The listing builds one solid part. Answer for the finished solid, in the listing's coordinates (mm). Coordinates: 2 decimals unless noted, no trailing zeros. Order: outer loops, then holes, each group sorted by start corner. A loop starts at its lowest first (then second) coordinate and runs counter-clockwise, first axis right, second up. Notation, with made-up numbers: (-28.5, -26.5) -> (-15.5, -26.5) arc R24 ccw to (-15.5, -2.5) -> close; hole circle Ø1 at (75, -1). An arc over 180 degrees is marked (long way). Return JSON: item names as keys, results as strings.
```python
from build123d import *

# Parameters (mm, degrees)
EXTRUDE_1_DEPTH          = 5
CUT_EXTRUDE_2_DEPTH      = 1
CUT_EXTRUDE_2_DEPTH_BACK = 6
CUT_EXTRUDE_3_REACH      = 7
CHAMFER_1_SIZE           = 5
CUT_EXTRUDE_6_DEPTH      = 1
CUT_EXTRUDE_6_DEPTH_BACK = 6
CHAMFER_2_SIZE           = 5
SKETCH_6_R               = 2.1
CUT_EXTRUDE_7_DEPTH      = 5
FILLET_1_R               = 10
M3X0_5_1_D               = 2.5
M3X0_5_1_DEPTH           = 8.5
M3X0_5_1_TIP             = 0.751075774
M4X0_7_2_D               = 3.3
M4X0_7_2_DEPTH           = 11.5
M4X0_7_2_TIP             = 0.991420021


with BuildPart() as part:
    # 草圖1 → 填料-伸長1 (new body)
    with BuildSketch(Plane.XY):
        Polygon((150, 0), (75, 129.903810568), (-75, 129.903810568), (-150, 0), (-75, -129.903810568), (75, -129.903810568), align=None)
    extrude(amount=EXTRUDE_1_DEPTH)

    # 草圖3 → 除料-伸長2 (cut, two sides)
    with BuildSketch(Plane.XY.offset(5)) as cut_extrude_2_sk:
        Polygon((-774.886138932, 69.903810568), (-109.641016151, 69.903810568), (-89.641016151, 69.903810568), (-89.641016151, 54.903810568), (0, 54.903810568), (0, 69.903810568), (109.641016151, 69.903810568), (774.886138932, 69.903810568), (774.886138932, 1400.394056128), (-774.886138932, 1400.394056128), align=None)
    extrude(amount=CUT_EXTRUDE_2_DEPTH, mode=Mode.SUBTRACT)
    extrude(cut_extrude_2_sk.sketch, amount=-CUT_EXTRUDE_2_DEPTH_BACK, mode=Mode.SUBTRACT)

    # 草圖4 → 除料-伸長3 (cut, up to next)
    with BuildSketch(Plane.XY.offset(5), mode=Mode.PRIVATE) as cut_extrude_3_sk1:
        Polygon((30, 0), (15, 25.980762114), (-15, 25.980762114), (-30, 0), (-15, -25.980762114), (15, -25.980762114), align=None)
    cut_extrude_3_tool1 = extrude(cut_extrude_3_sk1.sketch, amount=-CUT_EXTRUDE_3_REACH, mode=Mode.PRIVATE) & part.part
    add(cut_extrude_3_tool1.solids().sort_by_distance((0, 0, 5))[0], mode=Mode.SUBTRACT)

    # 導角1
    chamfer_1_edges = [part.edges().sort_by_distance(p)[0] for p in [
        (-89.641016151, 69.903810568, 2.5),
        (0, 69.903810568, 2.5),
    ]]
    chamfer(chamfer_1_edges, length=CHAMFER_1_SIZE)

    # 草圖5 → 除料-伸長6 (cut, two sides)
    with BuildSketch(Plane.XY.offset(5)) as cut_extrude_6_sk:
        Polygon((-692.345987228, -104.903810568), (-89.43375673, -104.903810568), (-30, -104.903810568), (-30, -64.903810568), (30, -64.903810568), (30, -104.903810568), (89.43375673, -104.903810568), (692.345987228, -104.903810568), (692.345987228, -1310.728271565), (-692.345987228, -1310.728271565), align=None)
    extrude(amount=CUT_EXTRUDE_6_DEPTH, mode=Mode.SUBTRACT)
    extrude(cut_extrude_6_sk.sketch, amount=-CUT_EXTRUDE_6_DEPTH_BACK, mode=Mode.SUBTRACT)

    # 導角2
    chamfer_2_edges = [part.edges().sort_by_distance(p)[0] for p in [
        (30, -104.903810568, 2.5),
        (-30, -104.903810568, 2.5),
        (-30, -64.903810568, 2.5),
        (30, -64.903810568, 2.5),
    ]]
    chamfer(chamfer_2_edges, length=CHAMFER_2_SIZE)

    # 草圖6 → 除料-伸長7 (cut)
    with BuildSketch(Plane.XY.offset(5)):
        with Locations((-50, -90)):
            Circle(SKETCH_6_R)
        with Locations((-120, 10)):
            Circle(SKETCH_6_R)
        with Locations((-60, 30)):
            Circle(SKETCH_6_R)
        with Locations((-20, -50)):
            Circle(SKETCH_6_R)
    cut_extrude_7 = extrude(amount=-CUT_EXTRUDE_7_DEPTH, mode=Mode.SUBTRACT)

    # 鏡射1: 除料-伸長7 across plane
    add(cut_extrude_7.mirror(Plane(origin=(0, 0, 0), x_dir=(0, 0, 1), z_dir=(1, 0, 0))), mode=Mode.SUBTRACT)

    # 圓角1
    fillet_1_edges = [part.edges().sort_by_distance(p)[0] for p in [
        (-150, 0, 2.5),
        (150, 0, 2.5),
        (109.641016151, 69.903810568, 2.5),
        (-109.641016151, 69.903810568, 2.5),
        (-89.43375673, -104.903810568, 2.5),
        (89.43375673, -104.903810568, 2.5),
    ]]
    fillet(fillet_1_edges, radius=FILLET_1_R)

    # M3x0.5 螺紋孔1
    with Locations(Plane.XY.offset(5)):
        with Locations((95, 15.096189432), (75, -54.903810568), (75, 15.096189432), (95, -54.903810568)):
            Hole(M3X0_5_1_D / 2, depth=M3X0_5_1_DEPTH)
            with Locations((0, 0, -(M3X0_5_1_DEPTH + M3X0_5_1_TIP / 2))):  # 118° drill point
                Cone(0, M3X0_5_1_D / 2, M3X0_5_1_TIP, mode=Mode.SUBTRACT)

    # M4x0.7 螺紋孔2
    with Locations(Plane.XY.offset(5)):
        with Locations((25, 35), (-25, -35), (-25, 35), (25, -35), (-35, 0), (35, 0)):
            Hole(M4X0_7_2_D / 2, depth=M4X0_7_2_DEPTH)
            with Locations((0, 0, -(M4X0_7_2_DEPTH + M4X0_7_2_TIP / 2))):  # 118° drill point
                Cone(0, M4X0_7_2_D / 2, M4X0_7_2_TIP, mode=Mode.SUBTRACT)


solid = part.part
```
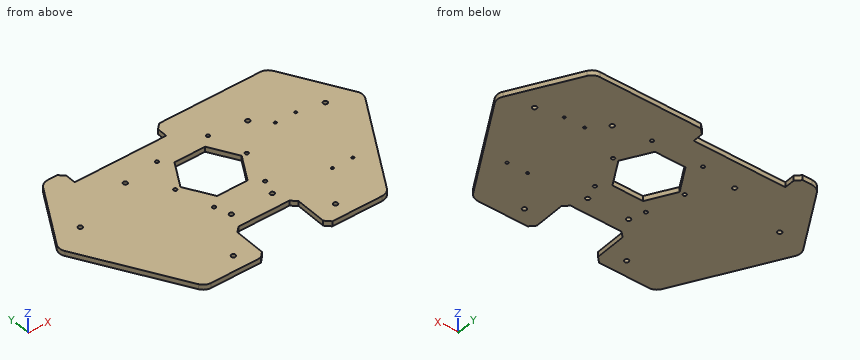
Item 1: The part is cut by section B-B on z = 2.6. Count the separate pieces of the cut face and the enclosed holes in it, plus the area to 3 significant figures.
Answer list:
{"separate pieces": "1", "enclosed holes": "19", "area": "36,900 mm2"}
Item 2: The part is cut by section A-A on x = -55. Determine the outline of the cut face in (y, z), plus the area to 3 significant figures.
Answer list:
{"outline": "(-104.9, 0) -> (54.9, 0) -> (54.9, 5) -> (-104.9, 5) -> close", "area": "799 mm2"}
Item 3: Flat-ended cylindrical pins translate along their axes: pin 1 (3 mm diameter, centred on x = 25, y = 35, fed in from -Z); pin 2 (2 mm diameter, centred on y = -17, z = 1, fed in from +X); pin 3 (1.5 mm diameter, centred on x = 7, z = 1.5, fed in from -Y); pin 4 (2 mm diameter, centred on y = -4, z = 4, fed in from -X). Find the tip coordinate at first contact, or state that the pin passes through.
Answer list:
{"pin 1": "through", "pin 2": "x = 140.76", "pin 3": "y = -64.9", "pin 4": "x = -147.99"}
Item 4: The part is cut by section C-C on y = 45. Determine the outline of the cut face in (x, z), plus the area to 3 significant figures.
Answer list:
{"outline": "(-124.02, 0) -> (124.02, 0) -> (124.02, 5) -> (-124.02, 5) -> close", "area": "1,240 mm2"}
Item 5: Find the intervals of material crossed by probe 1 along X at (y, z) = (33.5, 4.5); probe 2 along Y at (x, z) = (50, 2.65); probe 3 along Y at (x, z) = (-25, 2.2), in increasing order.
Answer list:
{"probe 1": "-130.66 to -25.69, -24.31 to 24.31, 25.69 to 130.66", "probe 2": "-104.9 to -92.1, -87.9 to 69.9", "probe 3": "-64.9 to -36.65, -33.35 to -8.66, 8.66 to 33.35, 36.65 to 54.9"}
